from build123d import *

# Parameters (mm, degrees)
SKETCH003_W     = 60
SKETCH003_H     = 80
PAD_DEPTH       = 2.5
SKETCH_W        = 43
SKETCH_H        = 60.3
POCKET_DEPTH    = 5
SKETCH004_W     = 60
SKETCH004_H     = 80
SKETCH004_W_2   = 56
SKETCH004_H_2   = 76
PAD001_DEPTH    = 2
SKETCH005_W     = 7.2
SKETCH005_H     = 4
POCKET001_DEPTH = 5
FILLET_R        = 2
FILLET001_R     = 1
FILLET002_R     = 1
FILLET003_R     = 2
FILLET004_R     = 0.5
FILLET005_R     = 1.1


with BuildPart() as part:
    # Sketch003 → Pad (new body)
    with BuildSketch(Plane.XY):
        with Locations((30, 40)):
            Rectangle(SKETCH003_W, SKETCH003_H)
    extrude(amount=PAD_DEPTH)

    # Sketch (on Face6 of Pad) → Pocket (cut)
    with BuildSketch(Plane.XY.offset(2.5)):
        with Locations((30, 41.15)):
            Rectangle(SKETCH_W, SKETCH_H)
    extrude(amount=-POCKET_DEPTH, mode=Mode.SUBTRACT)

    # Sketch004 (on Face4 of Pocket) → Pad001 (join)
    with BuildSketch(Plane(origin=(0, 0, 0), x_dir=(1, 0, 0), z_dir=(0, 0, -1))):
        with Locations((30, -40)):
            Rectangle(SKETCH004_W, SKETCH004_H)
        with Locations((30, -40)):
            Rectangle(SKETCH004_W_2, SKETCH004_H_2, mode=Mode.SUBTRACT)
    extrude(amount=PAD001_DEPTH)

    # Sketch005 (on Face7 of Pad001) → Pocket001 (cut)
    with BuildSketch(Plane.XY.offset(2.5)):
        with Locations((27.6, 6)):
            Rectangle(SKETCH005_W, SKETCH005_H)
    extrude(amount=-POCKET001_DEPTH, mode=Mode.SUBTRACT)

    # Fillet
    fillet_edges = [part.edges().sort_by_distance(p)[0] for p in [
        (60, 0, 0.25),
        (0, 0, 0.25),
        (0, 80, 0.25),
        (60, 80, 0.25),
    ]]
    fillet(fillet_edges, radius=FILLET_R)

    # Fillet001
    fillet001_edges = [part.edges().sort_by_distance(p)[0] for p in [
        (30, 11, 2.5),
        (8.5, 41.15, 2.5),
        (30, 71.3, 2.5),
        (51.5, 41.15, 2.5),
    ]]
    fillet(fillet001_edges, radius=FILLET001_R)

    # Fillet002
    fillet002_edges = [part.edges().sort_by_distance(p)[0] for p in [
        (27.6, 4, 2.5),
        (24, 6, 2.5),
        (27.6, 8, 2.5),
        (31.2, 6, 2.5),
    ]]
    fillet(fillet002_edges, radius=FILLET002_R)

    # Fillet003
    fillet003_edges = [part.edges().sort_by_distance(p)[0] for p in [
        (30, 0, 2.5),
        (59.414214, 0.585786, 2.5),
        (60, 40, 2.5),
        (0.585786, 0.585786, 2.5),
        (0, 40, 2.5),
        (59.414214, 79.414214, 2.5),
        (30, 80, 2.5),
        (0.585786, 79.414214, 2.5),
    ]]
    fillet(fillet003_edges, radius=FILLET003_R)

    # Fillet004
    fillet004_edges = [part.edges().sort_by_distance(p)[0] for p in [
        (30, 2, -2),
        (58, 40, -2),
        (30, 78, -2),
        (2, 40, -2),
    ]]
    fillet(fillet004_edges, radius=FILLET004_R)

    # Fillet005
    fillet005_edges = [part.edges().sort_by_distance(p)[0] for p in [
        (2, 2, -0.75),
        (58, 2, -0.75),
        (2, 78, -0.75),
        (58, 78, -0.75),
    ]]
    fillet(fillet005_edges, radius=FILLET005_R)


solid = part.part
The listing builds one solid part. Answer for the finished solid, in the listing's coordinates (mm). Coordinates: 2 decimals unless noted, no trailing zeros. Loops run counter-clockwise (first coordinate to the right, second up) from the corner with the lowest first, then second, coordinate; pieces in that order, holes last.
1) Find section D-D on y = 74. Write down the section's boundary in (x, z), then the cut area to 3 significant figures.
2) Flat-ended cylindrical pins translate along their axes: pin 1 Ø0.8 at (y, z) = (6.5, 1) entering from +X; pin 2 Ø2 at (x, y) = (7, 50) entering from -Z. Find the tip coordinate at first contact, or state that the pin passes through.
3) Find section B-B on x = 26. Write down the section's boundary in (y, z), then the cut area to 3 significant figures.
4) Find the intervals of material crossed by L1, parallel to X at y = 19, z = -0.7; L2, parallel to Y at x = 21.5, z = 0.45; L3, parallel to X at y = 6, z = 0.6, in increasing order.
5) Find section C-C on x = 20. Write down the section's boundary in (y, z).
6) Determine the mould class of faces 1 (the face through (29.61, 79.4, 1.93)), 2 (the face through (5, 41, 0)), 3 (the face through (59.4, 0.57, -0.73)) for opening direction X: pulls with the +X half, pulls with the -X half, needs draft (parallel to the pull), parting line crosses it, or undercut.
7) Find section A-A on y = 59. Write down the section's boundary in (x, z), then the cut area to 3 significant figures.
Values:
1. outline: (0, -2) - (1.5, -2) arc R0.5 ccw to (2, -1.5) - (2, 0) - (58, 0) - (58, -1.5) arc R0.5 ccw to (58.5, -2) - (60, -2) - (60, 0.5) arc R2 ccw to (58, 2.5) - (2, 2.5) arc R2 ccw to (0, 0.5) - close
1. area: 156 mm2
2. pin 1: stops at x = 60
2. pin 2: stops at z = 0
3. outline: (0, -2) - (1.5, -2) arc R0.5 ccw to (2, -1.5) - (2, 0) - (4, 0) - (4, 1.5) arc R1 ccw to (3, 2.5) - (2, 2.5) arc R2 ccw to (0, 0.5) - close; (8, 0) - (11, 0) - (11, 1.5) arc R1 ccw to (10, 2.5) - (9, 2.5) arc R1 ccw to (8, 1.5) - close; (71.3, 0) - (78, 0) - (78, -1.5) arc R0.5 ccw to (78.5, -2) - (80, -2) - (80, 0.5) arc R2 ccw to (78, 2.5) - (72.3, 2.5) arc R1 ccw to (71.3, 1.5) - close
3. area: 44.6 mm2
4. L1: x = 0 to 2, 58 to 60
4. L2: y = 0 to 11, 71.3 to 80
4. L3: x = 0 to 24, 31.2 to 60
5. outline: (0, -2) - (1.5, -2) arc R0.5 ccw to (2, -1.5) - (2, 0) - (11, 0) - (11, 1.5) arc R1 ccw to (10, 2.5) - (2, 2.5) arc R2 ccw to (0, 0.5) - close; (71.3, 0) - (78, 0) - (78, -1.5) arc R0.5 ccw to (78.5, -2) - (80, -2) - (80, 0.5) arc R2 ccw to (78, 2.5) - (72.3, 2.5) arc R1 ccw to (71.3, 1.5) - close
6. face 1: needs draft
6. face 2: undercut
6. face 3: pulls with the +X half
7. outline: (0, -2) - (1.5, -2) arc R0.5 ccw to (2, -1.5) - (2, 0) - (8.5, 0) - (8.5, 1.5) arc R1 ccw to (7.5, 2.5) - (2, 2.5) arc R2 ccw to (0, 0.5) - close; (51.5, 0) - (58, 0) - (58, -1.5) arc R0.5 ccw to (58.5, -2) - (60, -2) - (60, 0.5) arc R2 ccw to (58, 2.5) - (52.5, 2.5) arc R1 ccw to (51.5, 1.5) - close
7. area: 48.2 mm2
